Here's the drawing with two shaded views (mm, measured from the low corner). I have some questions. A direction names the side the tool comes from. Give positions to 0.01 mm unless a question says otherwise; leave off trailing zeros. Loops run counter-clockwise (first coordinate to the right, second up) from the corner with the lowest first, then second, coordinate; pieces in that order, holes last. Notation, with made-up numbers: (-38.75, -22) -> (11.25, -22) arc R18 cw to (11.25, -4) -> close; hole circle Ø6 at (68.5, 27). An arc over 180 degrees is marked (long way). Write each question's results on one line, items separated by ' | '. Start each with the question number.
Q1. If we section it at C-C, the plane z = 3.1: List the corners of the cut face in (x, y) for me (1 decimal).
Q2. If I drill on line 1 along X through (y, z) = (76, 2.5); line 2 along Y through (x, z) = (10, 3.5) (1 decimal); line 3 along X through (y, z) = (51.5, 3.25), over which ranges is the centre line in solid material (lowest first)?
Q3. If we section it at A-A, the plane y = 63.5: List the corners of the cut face in (x, z) for me.
Q4. If we section it at D-D, the plane x = 24: List the corners of the cut face in (y, z) for me.
Q5. Will these pins go through, and if not, where does the flat tip stop? P1, Ø1.2, axis at x = 7.5, y = 82.04, coming from the -Z side; P2, Ø1.5, axis at y = 72, z = 2, coming from the +X side.
Q6. If we section it at B-B, the plane x = 4.5: List the corners of the cut face in (y, z) for me (1 decimal).
Q7. Which directions (+Z, -Z, +X, -X, +Y, -Y) give clear straight access to the entire face, cutting with the end or side of a thin tool? Please do the marked faces 1, 2 and 3.
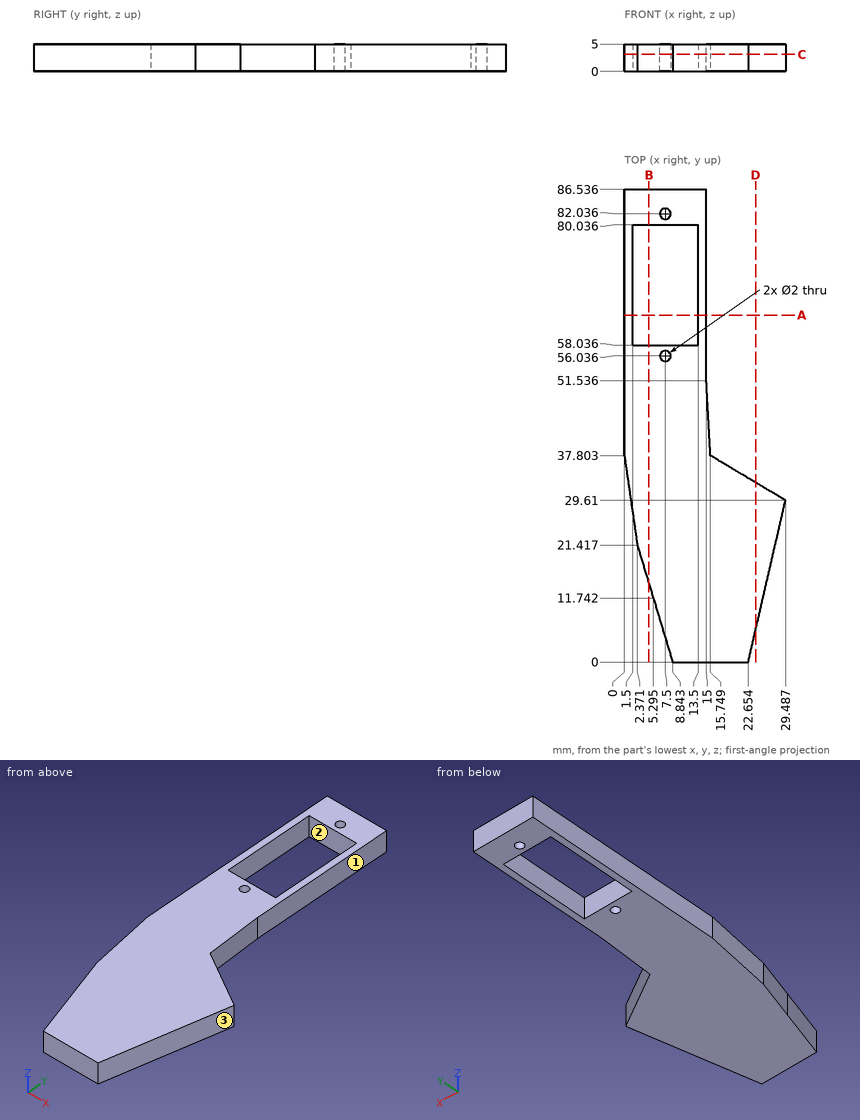
Final values:
1) outline: (0, 37.8) -> (2.4, 21.4) -> (8.8, 0) -> (22.7, 0) -> (29.5, 29.6) -> (15.7, 37.8) -> (15, 51.5) -> (15, 86.5) -> (0, 86.5) -> close; hole (1.5, 58) -> (13.5, 58) -> (13.5, 80) -> (1.5, 80) -> close; hole circle Ø2 at (7.5, 56); hole circle Ø2 at (7.5, 82)
2) line 1: x = 0 to 1.5, 13.5 to 15 | line 2: y = 0 to 58, 80 to 86.5 | line 3: x = 0 to 15
3) outline: (0, 0) -> (1.5, 0) -> (1.5, 5) -> (0, 5) -> close; (13.5, 0) -> (15, 0) -> (15, 5) -> (13.5, 5) -> close
4) outline: (5.83, 0) -> (32.88, 0) -> (32.88, 5) -> (5.83, 5) -> close
5) P1: passes through | P2: stops at x = 15
6) outline: (14.4, 0) -> (58, 0) -> (58, 5) -> (14.4, 5) -> close; (80, 0) -> (86.5, 0) -> (86.5, 5) -> (80, 5) -> close
7) face 1: +Z, -Z, +X, +Y | face 2: +Z, -Z | face 3: +Z, -Z, +X, -Y
